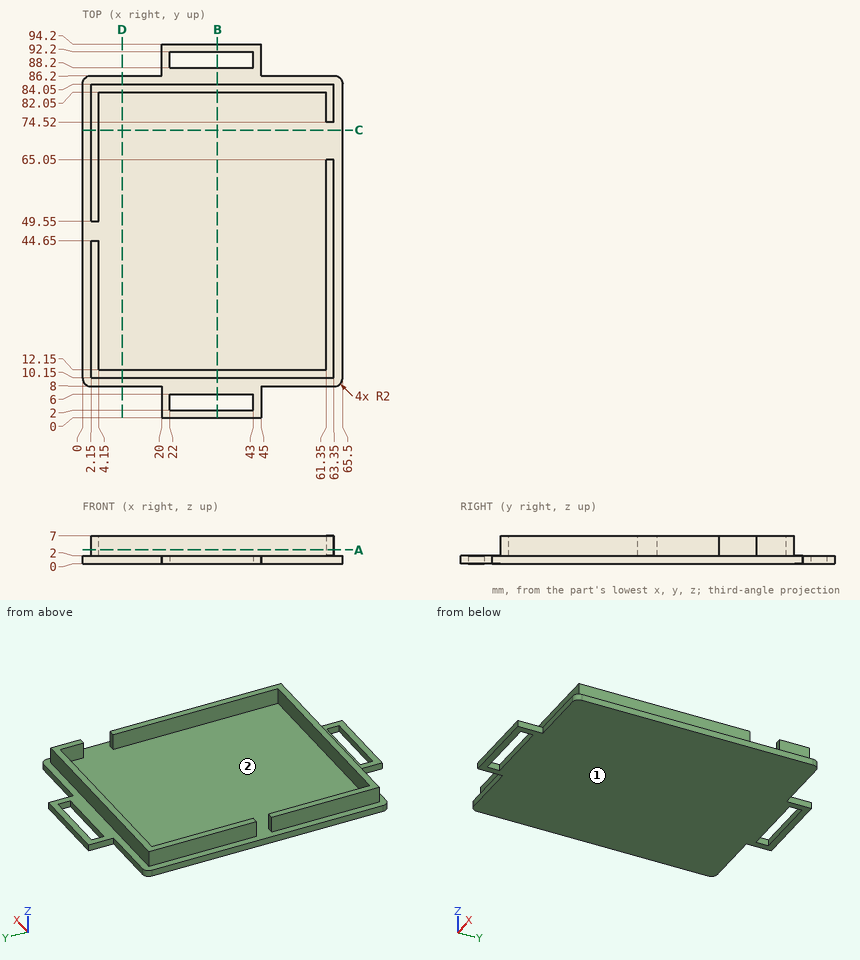
The figure shows three views and two pictorial views of one solid part (mm, origin at its lowest corner). Answer the questions. Give positions to 0.01 mm unless a question says otherwise; leave off trailing zeros. Loops run counter-clockwise (first coordinate to the right, second up) from the corner with the lowest first, then second, coordinate; pieces in that order, holes last. Notation, with made-up numbers: (-23.75, -0.75) - (21.25, -0.75) arc R10 cw to (21.25, 11.25) - close; hole circle Ø6 at (-7, -8.75). An arc over 180 degrees is marked (long way). Answer in a Markdown table with one row per item.
(1) Consider L1, parallel to Y at x = 26.5, z = 1.25; L2, parallel to Y at x = 43, z = 3.75; L3, parallel to X at y = 26, z = 5.75. Determine where each line is inside the solid, lowest interval first. Write a range as [from, to].
Results list:
| item | result |
|---|---|
| L1 | y = [0, 2], [6, 88.2], [92.2, 94.2] |
| L2 | y = [10.15, 12.15], [82.05, 84.05] |
| L3 | x = [2.15, 4.15], [61.35, 63.35] |
(2) Section C-C (y = 72.5) is taken. Give the vertices of the cut face in (x, z), and give its area (3 significant figures).
Results list:
| item | result |
|---|---|
| outline | (0, 0) - (65.5, 0) - (65.5, 2) - (4.15, 2) - (4.15, 7) - (2.15, 7) - (2.15, 2) - (0, 2) - close |
| area | 141 mm² |
(3) Section D-D (x = 10) is taken. Give the vertices of the cut face in (y, z).
Results list:
| item | result |
|---|---|
| outline | (8, 0) - (86.2, 0) - (86.2, 2) - (84.05, 2) - (84.05, 7) - (82.05, 7) - (82.05, 2) - (12.15, 2) - (12.15, 7) - (10.15, 7) - (10.15, 2) - (8, 2) - close |
(4) Section B-B (x = 34) is taken. Give the vertices of the cut face in (y, z).
Results list:
| item | result |
|---|---|
| outline | (0, 0) - (2, 0) - (2, 2) - (0, 2) - close; (6, 0) - (88.2, 0) - (88.2, 2) - (84.05, 2) - (84.05, 7) - (82.05, 7) - (82.05, 2) - (12.15, 2) - (12.15, 7) - (10.15, 7) - (10.15, 2) - (6, 2) - close; (92.2, 0) - (94.2, 0) - (94.2, 2) - (92.2, 2) - close |
(5) Flat-ended cylindrical pins translate along their axes: pin 1 Ø1.5 at (x, y) = (27, 64.5) entering from +Z; pin 2 Ø1.6 at (y, z) = (4, 1.5) entering from -X; pin 3 Ø1.5 at (y, z) = (49.5, 4.5) entering from +X. Find the tip coordinate at first contact, or state that the pin passes through.
Results list:
| item | result |
|---|---|
| pin 1 | stops at z = 2 |
| pin 2 | stops at x = 20 |
| pin 3 | stops at x = 63.35 |
(6) For a pull along X with two mould halves and no side action, classify the marked faces 1 and 2 as pulls with the +X half, pulls with the -X half, needs draft (parallel to the pull), parting line crosses it, or undercut.
Results list:
| item | result |
|---|---|
| face 1 | needs draft |
| face 2 | undercut |
(7) Section A-A (z = 3.5) is taken. Give the vertices of the cut face in (x, y).
Results list:
| item | result |
|---|---|
| outline | (2.15, 10.15) - (63.35, 10.15) - (63.35, 65.05) - (61.35, 65.05) - (61.35, 12.15) - (4.15, 12.15) - (4.15, 44.65) - (2.15, 44.65) - close; (2.15, 49.55) - (4.15, 49.55) - (4.15, 82.05) - (61.35, 82.05) - (61.35, 74.52) - (63.35, 74.52) - (63.35, 84.05) - (2.15, 84.05) - close |
